```python
from build123d import *

# Parameters (mm, degrees)
BOSS_EXTRUDE1_DEPTH = 190
SKETCH3_W           = 10
SKETCH3_H           = 170
CUT_EXTRUDE2_DEPTH  = 20
SKETCH4_W           = 170
SKETCH4_H           = 10
CUT_EXTRUDE3_DEPTH  = 20
SKETCH5_R           = 2.75
CUT_EXTRUDE4_DEPTH  = 10
SKETCH6_W           = 5
SKETCH6_H           = 20
CUT_EXTRUDE5_DEPTH  = 5
BOSS_EXTRUDE2_REACH = 195.391
SKETCH9_R           = 2.75
SKETCH9_R_2         = 2.5
SKETCH10_R          = 2.5
CUT_EXTRUDE6_DEPTH  = 194.390796058
SKETCH11_W          = 5
SKETCH11_H          = 20
CUT_EXTRUDE7_DEPTH  = 3
SKETCH12_R          = 2
CUT_EXTRUDE8_DEPTH  = 193.613602843


with BuildPart() as part:
    # Sketch2 → Boss-Extrude1 (new body)
    with BuildSketch(Plane.XY):
        Polygon((0, 0), (0, 10), (10, 10), (10, 30), (20, 30), (20, 0), align=None)
    extrude(amount=BOSS_EXTRUDE1_DEPTH)

    # Sketch3 → Cut-Extrude2 (cut)
    with BuildSketch(Plane.XZ):
        with Locations((15, 105)):
            Rectangle(SKETCH3_W, SKETCH3_H)
    extrude(amount=-CUT_EXTRUDE2_DEPTH, mode=Mode.SUBTRACT)

    # Sketch4 → Cut-Extrude3 (cut)
    with BuildSketch(Plane(origin=(10, 0, 0), x_dir=(0, 0, -1), z_dir=(1, 0, 0))):
        with Locations((-105, 5)):
            Rectangle(SKETCH4_W, SKETCH4_H)
    extrude(amount=-CUT_EXTRUDE3_DEPTH, mode=Mode.SUBTRACT)

    # Sketch5 → Cut-Extrude4 (cut)
    with BuildSketch(Plane.ZY):
        with Locations((10, 5)):
            Circle(SKETCH5_R)
    extrude(amount=-CUT_EXTRUDE4_DEPTH, mode=Mode.SUBTRACT)

    # Sketch6 → Cut-Extrude5 (cut)
    with BuildSketch(Plane(origin=(0, 30, 0), x_dir=(1, 0, 0), z_dir=(0, 1, 0))):
        with Locations((15, -180)):
            Rectangle(SKETCH6_W, SKETCH6_H)
    extrude(amount=-CUT_EXTRUDE5_DEPTH, mode=Mode.SUBTRACT)

    # Sketch9 → Boss-Extrude2 (add, up to next)
    with BuildSketch(Plane.ZY, mode=Mode.PRIVATE) as boss_extrude2_sk1:
        with Locations((10, 5)):
            Circle(SKETCH9_R)
        with Locations((10, 5)):
            Circle(SKETCH9_R_2, mode=Mode.SUBTRACT)
    boss_extrude2_tool1 = extrude(boss_extrude2_sk1.sketch, amount=-BOSS_EXTRUDE2_REACH, mode=Mode.PRIVATE) - part.part
    add(boss_extrude2_tool1.solids().sort_by_distance((0, 5, 7.327782))[0])

    # Sketch10 → Cut-Extrude6 (cut, through all)
    with BuildSketch(Plane.ZY):
        with Locations((10, 5)):
            Circle(SKETCH10_R)
    extrude(amount=-CUT_EXTRUDE6_DEPTH, mode=Mode.SUBTRACT)

    # Sketch11 → Cut-Extrude7 (cut)
    with BuildSketch(Plane(origin=(0, 25, 0), x_dir=(1, 0, 0), z_dir=(0, 1, 0))):
        with Locations((15, -180)):
            Rectangle(SKETCH11_W, SKETCH11_H)
    extrude(amount=-CUT_EXTRUDE7_DEPTH, mode=Mode.SUBTRACT)

    # Sketch12 → Cut-Extrude8 (cut, through all)
    with BuildSketch(Plane.ZY.offset(-10)):
        with Locations((180, 25)):
            Circle(SKETCH12_R)
    extrude(amount=-CUT_EXTRUDE8_DEPTH, mode=Mode.SUBTRACT)


solid = part.part
```
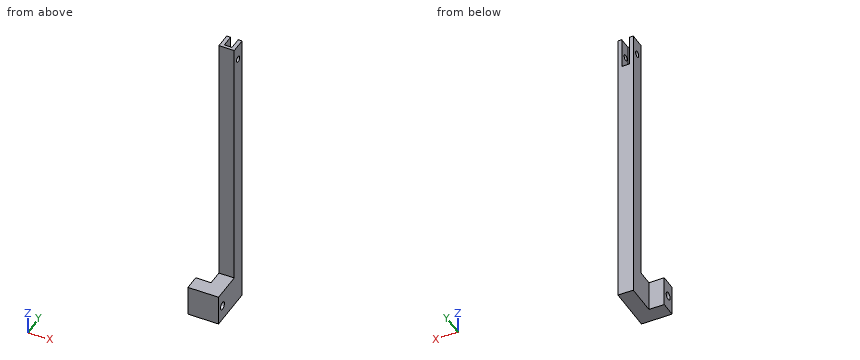
Design review of the part built by this model. Coordinates are the model's own, in mm. Coordinates: 2 decimals unless noted, no trailing zeros. Order: outer loops, then holes, each group sorted by start corner. A loop starts at its lowest first (then second) coordinate and runs counter-clockwise, first axis right, second up. Notation, with made-up numbers: (83, 24) - (112, 24) arc R20 cw to (112, 60) - close; hole circle Ø6 at (57, -32.75). An arc over 180 degrees is marked (long way). Answer in a Markdown table with one row per item.
(1) Clearance check with flat-ended pins moving along their axes: pin 1 (9 mm diameter, centred on y = 25.5, z = 183, fed in from -X); pin 2 (8 mm diameter, centred on x = 16.5, z = 87, fed in from -Y); pin 3 (3 mm diameter, centred on x = 6.5, z = 14.5, fed in from +Y). State where each tip first meets the part, or that it passes through.
Checked values:
| item | result |
|---|---|
| pin 1 | x = 10 |
| pin 2 | y = 20 |
| pin 3 | y = 10 |
(2) Consider section A-A on z = 10. State the section outline as (x, y) points, plus the area to 3 significant figures.
Checked values:
| item | result |
|---|---|
| outline | (0, 0) - (20, 0) - (20, 2.5) - (0, 2.5) - close; (0, 7.5) - (20, 7.5) - (20, 30) - (10, 30) - (10, 10) - (0, 10) - close |
| area | 300 mm^2 |
(3) Wall thickness on line 1 along Y through (x, z) = (11.2, 180); line 2 along Z through (x, y) = (12.75, 17.75); line 3 along Z through (x, y) = (1.75, 3.75): over which ranges is each line inside the solid? List them lowest first. Write a range as from..to.
Checked values:
| item | result |
|---|---|
| line 1 | 20..23, 27..30 |
| line 2 | 0..20 |
| line 3 | 0..7.83, 12.17..20 |
(4) Consider section B-B on y = 25. State the section outline as (x, z) points, plus the area to 3 significant figures.
Checked values:
| item | result |
|---|---|
| outline | (10, 0) - (20, 0) - (20, 178) - (17.5, 178) - (17.5, 170) - (12.5, 170) - (12.5, 178) - (10, 178) - close; (10, 182) - (12.5, 182) - (12.5, 190) - (10, 190) - close; (17.5, 182) - (20, 182) - (20, 190) - (17.5, 190) - close |
| area | 1,780 mm^2 |
(5) Consider section D-D on y = 5. State the section outline as (x, z) points.
Checked values:
| item | result |
|---|---|
| outline | (0, 0) - (20, 0) - (20, 7.5) - (0, 7.5) - close; (0, 12.5) - (20, 12.5) - (20, 20) - (0, 20) - close |
(6) Consider section C-C on z = 180. State the section outline as (x, y) points.
Checked values:
| item | result |
|---|---|
| outline | (10, 20) - (20, 20) - (20, 23) - (17.5, 23) - (17.5, 22) - (12.5, 22) - (12.5, 23) - (10, 23) - close; (10, 27) - (12.5, 27) - (12.5, 30) - (10, 30) - close; (17.5, 27) - (20, 27) - (20, 30) - (17.5, 30) - close |
